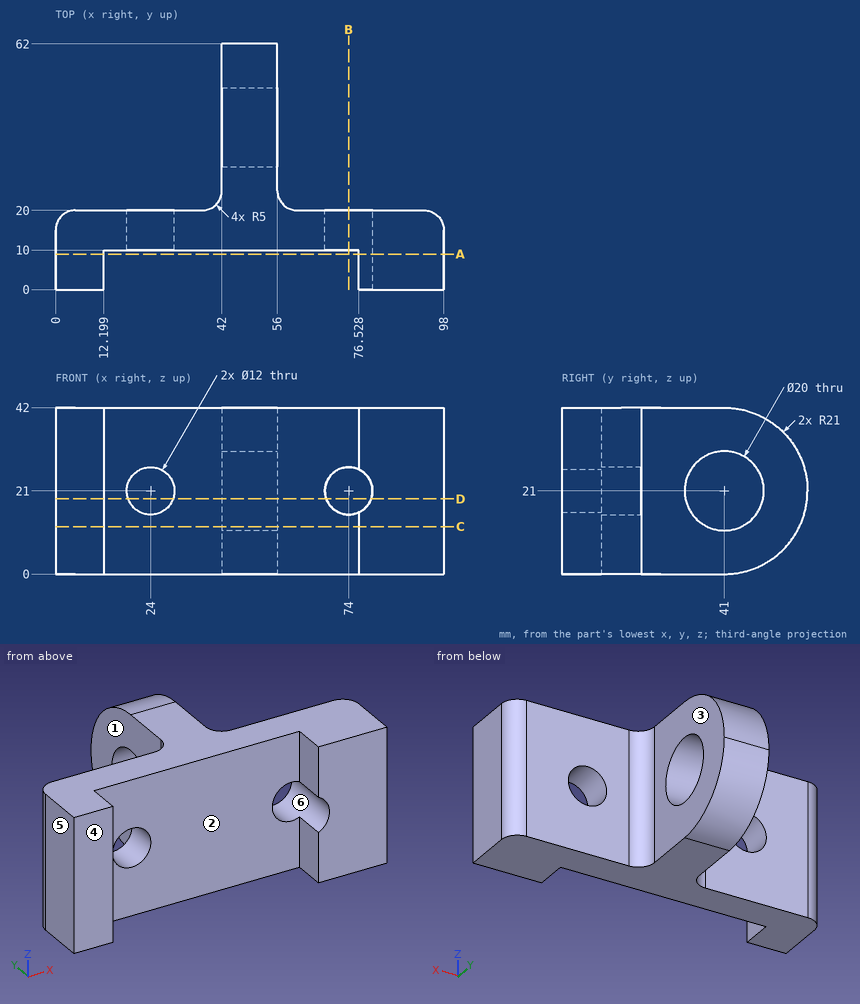
Geometry check sheet. Reference: drawing and pictorial views, mm from the part's lowest x, y, z. A direction names the side the tool comes from. Coordinates: 2 decimals unless noted, no trailing zeros. Loops run counter-clockwise (first coordinate to the right, second up) from the corner with the lowest first, then second, coordinate; pieces in that order, holes last. Notation, with made-up numbers: (80, 17) - (95, 17) arc R11 ccw to (95, 26) - close; hole circle Ø9 at (-21, -17). An arc over 180 degrees is marked (long way). Return JSON: item names as keys, results as strings.
1. Go/stop test with flat-tipped pins: pin 1 (4 mm diameter, centred on x = 44, z = 37, fed in from -Y); pin 2 (4 mm diameter, centred on y = 23.5, z = 26.5, fed in from +X); pin 3 (9.5 mm diameter, centred on x = 83.5, z = 17.5, fed in from +Y). Record where each tip stops, or that it passes through.
Established:
{"pin 1": "stops at y = 10", "pin 2": "stops at x = 57.43", "pin 3": "stops at y = 20"}
2. Section check C-C, the plane z = 12. Record the boundary of the cut face in (x, y), then the cut area to 3 significant figures.
Established:
{"outline": "(0, 0) - (12.2, 0) - (12.2, 10) - (76.53, 10) - (76.53, 0) - (98, 0) - (98, 15) arc R5 ccw to (93, 20) - (61, 20) arc R5 cw to (56, 25) - (56, 36.64) - (42, 36.64) - (42, 25) arc R5 cw to (37, 20) - (5, 20) arc R5 ccw to (0, 15) - close; (42, 45.36) - (56, 45.36) - (56, 59.97) - (42, 59.97) - close", "area": "1,750 mm2"}
3. Tool access check on the marked faces 1, 2 and 3. Record the directions out of +Z, -Z, +X, -X, +Y, -Y that give a thin tool (end or side, any length) a straight path to the whole face; none if there is none.
Established:
{"face 1": "+Z, -Z, -X, +Y", "face 2": "+Z, -Z, -Y", "face 3": "+Z, -Z, +X, +Y"}
4. Section check B-B, the plane x = 74. Record the boundary of the cut face in (y, z), then the cut area to 3 significant figures.
Established:
{"outline": "(10, 0) - (20, 0) - (20, 15) - (10, 15) - close; (10, 27) - (20, 27) - (20, 42) - (10, 42) - close", "area": "300 mm2"}
5. Thickness scan on L1, parallel to X at y = 13, z = 21; L2, parallel to Y at x = 47, z = 21; L3, parallel to X at y = 5.5, z = 32. Record the ranges inside material, lowest first.
Established:
{"L1": "x = 0 to 18, 30 to 68, 80 to 98", "L2": "y = 10 to 31, 51 to 62", "L3": "x = 0 to 12.2, 76.53 to 98"}
6. Section check D-D, the plane z = 19. Record the boundary of the cut face in (x, y), then the cut area to 3 significant figures.
Established:
{"outline": "(0, 0) - (12.2, 0) - (12.2, 10) - (18.34, 10) - (18.34, 20) - (5, 20) arc R5 ccw to (0, 15) - close; (29.66, 10) - (68.34, 10) - (68.34, 20) - (61, 20) arc R5 cw to (56, 25) - (56, 31.2) - (42, 31.2) - (42, 25) arc R5 cw to (37, 20) - (29.66, 20) - close; (42, 50.8) - (56, 50.8) - (56, 61.9) - (42, 61.9) - close; (79.66, 0) - (98, 0) - (98, 15) arc R5 ccw to (93, 20) - (79.66, 20) - close", "area": "1,370 mm2"}
7. Section check A-A, the plane y = 9. Record the boundary of the cut face in (x, z).
Established:
{"outline": "(0, 0) - (12.2, 0) - (12.2, 42) - (0, 42) - close; (76.53, 0) - (98, 0) - (98, 42) - (76.53, 42) - (76.53, 26.44) arc R6 cw to (76.53, 15.56) - close"}
8. Mould release check, pull along X, two halves, no side actions. Record for the marked faces 4, 5 and 6: +X half, -X half, draft (parallel to the pull), parting line (faces both ways), or undercut.
Established:
{"face 4": "draft", "face 5": "-X half", "face 6": "undercut"}
